from build123d import *

# Parameters (mm, degrees)
F0_W     = 25
F0_H     = 32.5
F0_W_2   = 2.5
F1_DEPTH = 5
F2_DEPTH = 6
F3_DEPTH = 5
F4_R     = 0.99999


# Not quite as in the source:
# - a fillet or chamfer is up to 0.001 mm smaller than in the source, because OpenCascade refuses the exact size


with BuildPart() as f1:
    # F0 (on Top) → F1 (new body)
    with BuildSketch(Plane.XY):
        Rectangle(F0_W, F0_H)
        Polygon((-15, 16.25), (-12.5, 16.25), (12.5, 16.25), (15, 16.25), (15, 18.75), (-15, 18.75), align=None)
        with Locations((-13.75, 0)):
            Rectangle(F0_W_2, F0_H)
        Polygon((12.5, -16.25), (-12.5, -16.25), (-15, -16.25), (-15, -18.75), (15, -18.75), (15, -16.25), align=None)
        with Locations((13.75, 0)):
            Rectangle(F0_W_2, F0_H)
    extrude(amount=F1_DEPTH)

    # F0 (on Top) → F2 (join)
    with BuildSketch(Plane.XY):
        Polygon((-15, 16.25), (-12.5, 16.25), (12.5, 16.25), (15, 16.25), (15, 18.75), (-15, 18.75), align=None)
        with Locations((-13.75, 0)):
            Rectangle(F0_W_2, F0_H)
        Polygon((12.5, -16.25), (-12.5, -16.25), (-15, -16.25), (-15, -18.75), (15, -18.75), (15, -16.25), align=None)
        with Locations((13.75, 0)):
            Rectangle(F0_W_2, F0_H)
    extrude(amount=F2_DEPTH)

    # F0 (on Top) → F3 (join)
    with BuildSketch(Plane.XY):
        Polygon((12.5, -16.25), (-12.5, -16.25), (-15, -16.25), (-15, -18.75), (15, -18.75), (15, -16.25), align=None)
        Polygon((-15, 16.25), (-12.5, 16.25), (12.5, 16.25), (15, 16.25), (15, 18.75), (-15, 18.75), align=None)
    extrude(amount=-F3_DEPTH)

    # F4 (radius 1 in the source; OpenCascade refuses exactly that, so slightly less here)
    f4_edges = [f1.edges().sort_by_distance(p)[0] for p in [
        (0, 16.25, -5),
        (15, 17.5, -5),
        (0, 18.75, -5),
        (-15, 17.5, -5),
        (-15, -17.5, -5),
        (0, -18.75, -5),
        (15, -17.5, -5),
        (0, -16.25, -5),
        (0, 16.25, 6),
        (12.5, 0, 6),
        (0, -16.25, 6),
        (-12.5, 0, 6),
        (0, 18.75, 6),
        (-15, 0, 6),
        (0, -18.75, 6),
        (15, 0, 6),
        (-15, -18.75, 0.5),
        (-15, -16.25, -2.5),
        (-15, 0, 0),
        (-15, 16.25, -2.5),
        (-15, 18.75, 0.5),
        (15, 18.75, 0.5),
        (15, -18.75, 0.5),
        (15, 16.25, -2.5),
        (15, 0, 0),
        (15, -16.25, -2.5),
    ]]
    fillet(f4_edges, radius=F4_R)


solid = f1.part
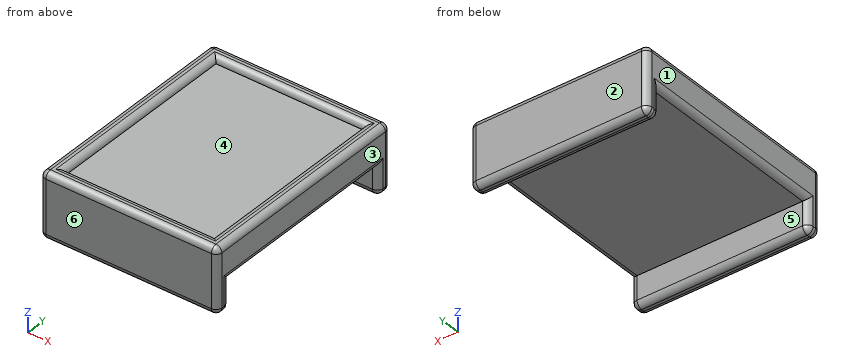
Work out the finished part from the listing and answer in its coordinate system (mm). Face numbers are marked on the shaded views. A direction names the side the tool comes from. Coordinates: 2 decimals unless noted, no trailing zeros. Write item = value, one per line.
1. Straight lines are drawn through the part: line 1 (Y direction, x = 13, z = -2.25); line 2 (Z direction, x = -2, y = 8); line 3 (Z direction, x = 13.5, y = 9). For each, find the intervals that lie inside material, in ascending order. Write a range as from..to.
Solution:
line_1 = -18.75..-16.25, 16.25..18.75
line_2 = 0..5
line_3 = 0..6
2. Flat-ended cylindrical pins translate along their axes: pin 1 (4 mm diameter, centred on x = 7, y = -13.5, fed in from +Z); pin 2 (6 mm diameter, centred on x = 11.5, y = -0.5, fed in from -Z). Find the tip coordinate at first contact, or state that the pin passes through.
Solution:
pin_1 = 5
pin_2 = 0
3. Determine the mould class of the marked faces 1, 2, 3 and 4 for opening direction X: released by +X, released by -X, zero draft, split by the parting line, or undercut.
Solution:
face_1 = released by -X
face_2 = zero draft
face_3 = released by +X
face_4 = undercut
4. For the marked faces 5 and 6, determine the directions among +Z, -Z, +X, -X, +Y, -Y from which every point of the face is accessible in a straight line to the end or side of a thin tool.
Solution:
face_5 = -Z, +X, -X
face_6 = +Z, -Z, +X, -X, -Y
